```python
from build123d import *

# Parameters (mm, degrees)
SKETCH1_W           = 5
SKETCH1_H           = 12
BOSS_EXTRUDE1_DEPTH = 10.95
SKETCH6_W           = 6.966027875
SKETCH6_H           = 1.5
BOSS_EXTRUDE2_DEPTH = 1
SKETCH4_W           = 10
SKETCH4_H           = 1.5
BOSS_EXTRUDE4_DEPTH = 1
SKETCH9_W           = 1.5
SKETCH9_H           = 17
BOSS_EXTRUDE5_DEPTH = 1
SKETCH10_W          = 1.5
SKETCH10_H          = 13
BOSS_EXTRUDE6_DEPTH = 1
SKETCH11_W          = 4.266730231
SKETCH11_H          = 1.5
BOSS_EXTRUDE7_DEPTH = 1


with BuildPart() as part:
    # Sketch1 → Boss-Extrude1 (new body)
    with BuildSketch(Plane.XY):
        Polygon((0, 0), (-10, 0), (-10, 15), (-3.033972125, 15), (0, 12), align=None)
        with Locations((-5.696428571, 7.758057491)):
            Rectangle(SKETCH1_W, SKETCH1_H, mode=Mode.SUBTRACT)
    extrude(amount=BOSS_EXTRUDE1_DEPTH)

    # Sketch6 → Boss-Extrude2 (add)
    with BuildSketch(Plane(origin=(0, 15, 0), x_dir=(1, 0, 0), z_dir=(0, 1, 0))):
        with Locations((-6.516986063, -8.120873767)):
            Rectangle(SKETCH6_W, SKETCH6_H)
    extrude(amount=BOSS_EXTRUDE2_DEPTH)

    # Sketch4 → Boss-Extrude4 (add)
    with BuildSketch(Plane.XZ):
        with Locations((-5, 8.120873767)):
            Rectangle(SKETCH4_W, SKETCH4_H)
    extrude(amount=BOSS_EXTRUDE4_DEPTH)

    # Sketch9 → Boss-Extrude5 (add)
    with BuildSketch(Plane.ZY.offset(10)):
        with Locations((8.120873767, 7.5)):
            Rectangle(SKETCH9_W, SKETCH9_H)
    extrude(amount=BOSS_EXTRUDE5_DEPTH)

    # Sketch10 → Boss-Extrude6 (add)
    with BuildSketch(Plane(origin=(0, 0, 0), x_dir=(0, 0, -1), z_dir=(1, 0, 0))):
        with Locations((-8.120873767, 5.5)):
            Rectangle(SKETCH10_W, SKETCH10_H)
    extrude(amount=BOSS_EXTRUDE6_DEPTH)

    # Sketch11 → Boss-Extrude7 (add)
    with BuildSketch(Plane(origin=(5.99961963, 6.067559573, 0), x_dir=(0.7110766234784633, -0.7031145251966195, 0), z_dir=(0.7031145251966195, 0.7110766234784633, 0))):
        with Locations((-10.570739418, -8.120873767)):
            Rectangle(SKETCH11_W, SKETCH11_H)
    extrude(amount=BOSS_EXTRUDE7_DEPTH)


solid = part.part
```
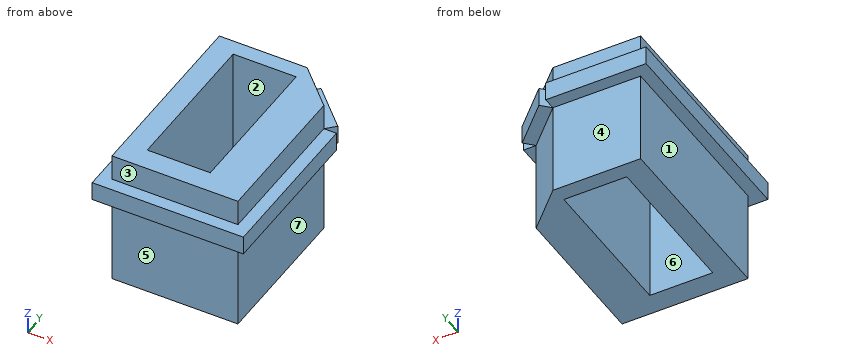
Geometry check sheet. Reference: the model listing, model coordinates, mm. Face numbers are marked on the shaded views. A direction names the side the tool comes from. Coordinates: 2 decimals unless noted, no trailing zeros. Loops run counter-clockwise (first coordinate to the right, second up) from the corner with the lowest first, then second, coordinate; pieces in that order, holes last.
Item 1: Sectioned sample at C-C, the plane z = 6.25. Record the boundary of the cut face in (x, y), then the cut area to 3 significant figures.
Item 2: Sectioned sample at D-D, the plane x = -9.25. Record the boundary of the cut face in (y, z), then the cut area to 3 significant figures.
Item 3: Thickness scan on line 1 (Y direction, x = -3.75, z = 5.75); line 2 (X direction, y = 11.5, z = 3); line 3 (X direction, y = 11.25, z = 8.25). Record the ranges inside material, lowest first.
Item 4: Release check for a two-part mould opening along X. For the marked faces 5, 6 and 7 record: released by +X, released by -X, zero draft, split by the parting line, or undercut.
Item 5: Sectioned sample at A-A, the plane x = -6.25. Record the boundary of the cut face in (y, z), then the cut area to 4 significant figures.
Item 6: Go/stop test with flat-tipped pins: pin 1 Ø3 at (x, y) = (-1, 15) entering from -Z; pin 2 Ø1 at (y, z) = (4, 10.5) entering from -X; pin 3 Ø0.8 at (y, z) = (15.5, 8) entering from +X; pin 4 Ø1 at (y, z) = (7.5, 10) entering from +X. Record where each tip stops, or that it passes through.
Item 7: Sectioned sample at B-B, the plane y = 4.75. Record the boundary of the cut face in (x, z).
Item 8: Access from +Z, -Z, +X, -X, +Y, -Y to the whole of each face (thin tool, end or side, straight path). Record for the marked faces 1, 2, 3 and 4.
Check result:
1. outline: (-10, 0) - (0, 0) - (0, 12) - (-3.03, 15) - (-10, 15) - close; hole (-8.2, 1.76) - (-3.2, 1.76) - (-3.2, 13.76) - (-8.2, 13.76) - close
1. area: 85.4 mm2
2. outline: (-1, 7.37) - (0, 7.37) - (0, 0) - (15, 0) - (15, 7.37) - (16, 7.37) - (16, 8.87) - (15, 8.87) - (15, 10.95) - (0, 10.95) - (0, 8.87) - (-1, 8.87) - close
2. area: 167 mm2
3. line 1: y = 0 to 1.76, 13.76 to 15
3. line 2: x = -10 to -8.2, -3.2 to 0
3. line 3: x = -11 to -8.2, -3.2 to 1
4. face 5: zero draft
4. face 6: undercut
4. face 7: released by +X
5. outline: (-1, 7.37) - (0, 7.37) - (0, 0) - (1.76, 0) - (1.76, 10.95) - (0, 10.95) - (0, 8.87) - (-1, 8.87) - close; (13.76, 0) - (15, 0) - (15, 7.37) - (16, 7.37) - (16, 8.87) - (15, 8.87) - (15, 10.95) - (13.76, 10.95) - close
5. area: 35.85 mm2
6. pin 1: stops at z = 0
6. pin 2: stops at x = -10
6. pin 3: stops at x = -1.71
6. pin 4: stops at x = 0
7. outline: (-11, 7.37) - (-10, 7.37) - (-10, 0) - (-8.2, 0) - (-8.2, 10.95) - (-10, 10.95) - (-10, 8.87) - (-11, 8.87) - close; (-3.2, 0) - (0, 0) - (0, 7.37) - (1, 7.37) - (1, 8.87) - (0, 8.87) - (0, 10.95) - (-3.2, 10.95) - close
8. face 1: -Z, -X, +Y, -Y
8. face 2: +Z, -Z
8. face 3: +Z, +X, -X, -Y
8. face 4: -Z, +X, -X, +Y
